from build123d import *

# Parameters (mm, degrees)
PROFILE_SKETCH1_R                    = 7.5
PROFILE_BOSS_EXTRUDE2_DEPTH          = 37.25987
FASTENINGHOLESKETCH3_R               = 2
FASTENINGHOLECUT_EXTRUDE8_DEPTH      = 56.995963358
LM8UUFASTENINGHOLESKETCH5_R          = 2
LM8UUFASTENINGHOLECUT_EXTRUDE9_DEPTH = 56.995963425


with BuildPart() as part:
    # Profile-Sketch1 → Profile-Boss-Extrude2 (new body)
    with BuildSketch(Plane(origin=(0, 0, 0), x_dir=(1, 0, 0), z_dir=(0, 1, 0))):
        with BuildLine():
            Line((-25, -21), (25, -21))
            Line((25, -21), (25, -15))
            Line((25, -15), (22.5, -15))
            ThreePointArc((22.5, -15), (15.428932188, -12.071067812), (12.5, -5))
            Line((12.5, -5), (12.5, 0))
            ThreePointArc((12.5, 0), (0, 12.5), (-12.5, 0))
            Line((-12.5, 0), (-12.5, -5))
            ThreePointArc((-12.5, -5), (-15.428932188, -12.071067812), (-22.5, -15))
            Line((-22.5, -15), (-25, -15))
            Line((-25, -15), (-25, -21))
        make_face()
        with Locations(Location((0, 0, 0), (0, 0, 270))):
            Circle(PROFILE_SKETCH1_R, mode=Mode.SUBTRACT)
    extrude(amount=PROFILE_BOSS_EXTRUDE2_DEPTH)

    # FasteningHoleSketch3 → FasteningHoleCut-Extrude8 (cut, through all)
    with BuildSketch(Plane.XY.offset(21)):
        with Locations((-17.0625, 29.32237)):
            Circle(FASTENINGHOLESKETCH3_R)
        with Locations((17.0625, 29.32237)):
            Circle(FASTENINGHOLESKETCH3_R)
    extrude(amount=-FASTENINGHOLECUT_EXTRUDE8_DEPTH, mode=Mode.SUBTRACT)

    # LM8UUFasteningHoleSketch5 → LM8UUFasteningHoleCut-Extrude9 (cut, through all)
    with BuildSketch(Plane.XY.offset(21)):
        with Locations((0, 12)):
            Circle(LM8UUFASTENINGHOLESKETCH5_R)
    extrude(amount=-LM8UUFASTENINGHOLECUT_EXTRUDE9_DEPTH, mode=Mode.SUBTRACT)


solid = part.part
Design review of the part built by this model. Coordinates are the model's own, in mm. A direction names the side the tool comes from. Give positions to 0.01 mm unless a question says otherwise; leave off trailing zeros. Order: outer loops, then holes, each group sorted by start corner. A loop starts at its lowest first (then second) coordinate and runs counter-clockwise, first axis right, second up. Notation, with made-up numbers: (-20, -33.5) - (-12, -33.5) arc R5 cw to (-12, -26.5) - close; hole circle Ø5 at (16.25, -21.75). An arc over 180 degrees is marked (long way). Use CSV: the item, a comma, the result in double quotes. Start each with the question number.
Q1. Draft analysis for pull direction Y (two halves, no side actions). For faces 1 (the face through (15.064, 29.41, 17.443)), 2 (the face through (-12.5, 18, 2)), 3 (the face through (0, 0, 8)), 4 (the face through (0, 37.26, 8)), state which applies: pulls with the +Y half, pulls with the -Y half, needs draft (parallel to the pull), parting line crosses it, or undercut.
Q2. Take a section at D-D (y = 5.5). State the section outline as (x, z) points, and give its area (3 significant figures).
Q3. Machinability: for faces 5 (the face through (-24, 18, 15)), 6 (the face through (12.5, 18, 3)), 7 (the face through (0.275, 18.369, -12.497)), which of the approach directions +Z, -Z, +X, -X, +Y, -Y give a long, thin tool a straight path to every point of the face, cutting with its end or side? Answer none if there is none.
Q4. For line 1 (X direction, y = 4, z = 0); line 2 (Y direction, x = 0, z = 9); line 3 (X direction, y = 21.5, z = -10), list the stretches that pass through material, from the lowest coordinate up.
Q5. Take a section at A-A (x = 0). State the section outline as (y, z) points.
Q6. Take a section at C-C (z = 3). State the section outline as (x, y) points, and give its area (3 significant figures).
Q7. For P1, Ø1, axis at y = 22.5, z = -2.5, coming from the -X side; P2, Ø19.5, axis at x = 0, z = 0, coming from the -Y side; P3, Ø1, axis at y = 24.5, z = 6.5, coming from the +X side; P4, Ø2, axis at x = -24, y = 22, coming from the -Z side, all flat-tipped, find the tip position at first contact; note any pin that passes through.
Q8. Take a section at B-B (y = 28.5). State the section outline as (x, z) points, and give its area (3 significant figures).
Calculated:
1,face 1,"undercut"
1,face 2,"needs draft"
1,face 3,"pulls with the -Y half"
1,face 4,"pulls with the +Y half"
2,outline,"(-25, 15) - (-22.5, 15) arc R10 cw to (-12.5, 5) - (-12.5, 0) arc R12.5 ccw to (12.5, 0) - (12.5, 5) arc R10 cw to (22.5, 15) - (25, 15) - (25, 21) - (-25, 21) - close; hole circle Ø15 at (0, 0)"
2,area,"787 mm²"
3,face 5,"-Z, -X, +Y, -Y"
3,face 6,"-Z, +X, +Y, -Y"
3,face 7,"-Z, +Y, -Y"
4,line 1,"x = -12.5 to -7.5, 7.5 to 12.5"
4,line 2,"y = 0 to 10, 14 to 37.26"
4,line 3,"x = -7.5 to 7.5"
5,outline,"(0, -12.5) - (10, -12.5) - (10, -7.5) - (0, -7.5) - close; (0, 7.5) - (10, 7.5) - (10, 21) - (0, 21) - close; (14, -12.5) - (37.26, -12.5) - (37.26, -7.5) - (14, -7.5) - close; (14, 7.5) - (37.26, 7.5) - (37.26, 21) - (14, 21) - close"
6,outline,"(-12.5, 0) - (-6.87, 0) - (-6.87, 37.26) - (-12.5, 37.26) - close; (6.87, 0) - (12.5, 0) - (12.5, 37.26) - (6.87, 37.26) - close"
6,area,"419 mm²"
7,P1,"stops at x = -12.34"
7,P2,"stops at y = 0"
7,P3,"stops at x = 12.7"
7,P4,"stops at z = 15"
8,outline,"(-25, 15) - (-22.5, 15) arc R10 cw to (-18.89, 14.32) - (-18.89, 21) - (-25, 21) - close; (-15.24, 11.88) arc R10 cw to (-12.5, 5) - (-12.5, 0) arc R12.5 ccw to (12.5, 0) - (12.5, 5) arc R10 cw to (15.24, 11.88) - (15.24, 21) - (-15.24, 21) - close; (18.89, 14.32) arc R10 cw to (22.5, 15) - (25, 15) - (25, 21) - (18.89, 21) - close; hole circle Ø15 at (0, 0)"
8,area,"730 mm²"
